Check sheet for the modelled part. Datum: model origin and axes. Units: mm. A direction names the side the tool comes from. Give positions to 0.01 mm unless a question says otherwise; leave off trailing zeros. Loops run counter-clockwise (first coordinate to the right, second up) from the corner with the lowest first, then second, coordinate; pieces in that order, holes last. Notation, with made-up numbers: (32, 24) -> (89, 24) arc R20 cw to (89, 51) -> close; hole circle Ø6 at (84, 15). An arc over 180 degrees is marked (long way). Write each question's results on one line, items separated by ' | '. Start each with the question number.
1. Mould release check, pull along X, two halves, no side actions. Record for faces 1 (the face through (-5, 3.25, 0)), 2 (the face through (-10.4, 3.6, 0)), 3 (the face through (-1.5, 0.07, -5.63)): +X half, -X half, draft (parallel to the pull), parting line (faces both ways), or undercut.
2. Cross-section at A-A on y = -2.25. Record the boundary of the cut face in (x, z), and give its area (3 significant figures).
3. Cross-section at C-C on x = -8.25. Record the boundary of the cut face in (y, z), and give its area (3 significant figures).
4. Gauge pin test, flat ends, axial feed: pin 1 Ø0.8 at (y, z) = (3.5, -2) entering from +X; pin 2 Ø0.8 at (x, z) = (1, -6) entering from +Y. Record the tip position at first contact, or that the pin passes through.
5. Cross-section at D-D on z = 3.5. Record the boundary of the cut face in (x, y).
6. Material ranges on L1, parallel to Z at x = -4.25, y = 1.75; L2, parallel to X at y = 0, z = 5.7; L3, parallel to Y at x = -6.5, z = -0.5, recorded low to high. Write a range as from..to.
7. Tool access check on faces 4 (the face through (-3, -1, -5.25)), 5 (the face through (0.1, 3.6, -0.1)), 6 (the face through (-3, 0, 6)). Record the directions out of +Z, -Z, +X, -X, +Y, -Y that give a thin tool (end or side, any length) a straight path to the whole face; none if there is none.
8. Cross-section at B-B on y = 0. Record the boundary of the cut face in (x, z).
from build123d import *

# Parameters (mm, degrees)
SKETCH1_R               = 1.5
BOSS_EXTRUDE1_DEPTH     = 6
FILLET1_R               = 1
CUT_EXTRUDE2_DEPTH      = 13.655433616
CUT_EXTRUDE2_DEPTH_BACK = 13.655433616
CUT_EXTRUDE3_DEPTH      = 16.748015748
CUT_EXTRUDE3_DEPTH_BACK = 3.5


with BuildPart() as part:
    # Sketch1 → Boss-Extrude1 (new, symmetric)
    with BuildSketch(Plane.XY):
        Polygon((-10.4, -3), (-0.7, -3), (-0.55, -4), (3.6, -3.7), (3.6, 4), (-10.4, 4), align=None)
        Circle(SKETCH1_R, mode=Mode.SUBTRACT)
    extrude(amount=BOSS_EXTRUDE1_DEPTH, both=True)

    # Fillet1
    fillet1_edges = [part.edges().sort_by_distance(p)[0] for p in [
        (-3.4, 4, -6),
        (-3.4, 4, 6),
    ]]
    fillet(fillet1_edges, radius=FILLET1_R)

    # Sketch2 → Cut-Extrude2 (cut, two sides: drawn at the far end of the back side and taken through both)
    with BuildSketch(Plane(origin=(0, 0, 0), x_dir=(0, 0, -1), z_dir=(1, 0, 0)).offset(-CUT_EXTRUDE2_DEPTH_BACK)):
        with BuildLine():
            Line((-5.25, 3), (-5.25, -4))
            Line((-5.25, -4), (5.25, -4))
            Line((5.25, -4), (5.25, 3))
            ThreePointArc((5.25, 3), (5.176776695, 3.176776695), (5, 3.25))
            Line((5, 3.25), (-5, 3.25))
            ThreePointArc((-5, 3.25), (-5.176776695, 3.176776695), (-5.25, 3))
        make_face()
    extrude(amount=CUT_EXTRUDE2_DEPTH + CUT_EXTRUDE2_DEPTH_BACK, mode=Mode.SUBTRACT)

    # Sketch3 → Cut-Extrude3 (cut, two sides: drawn at the far end of the back side and taken through both)
    with BuildSketch(Plane(origin=(3.6, 0, 0), x_dir=(0, 0, -1), z_dir=(1, 0, 0)).offset(-CUT_EXTRUDE3_DEPTH_BACK)):
        with BuildLine():
            Line((-5, 4), (5, 4))
            ThreePointArc((5, 4), (5.707106781, 3.707106781), (6, 3))
            Line((6, 3), (-6, 3))
            ThreePointArc((-6, 3), (-5.707106781, 3.707106781), (-5, 4))
        make_face()
    extrude(amount=CUT_EXTRUDE3_DEPTH + CUT_EXTRUDE3_DEPTH_BACK, mode=Mode.SUBTRACT)


solid = part.part
Geometry says:
1) face 1: draft | face 2: -X half | face 3: undercut
2) outline: (-10.4, -6) -> (3.6, -6) -> (3.6, -5.25) -> (-10.4, -5.25) -> close; (-10.4, 5.25) -> (3.6, 5.25) -> (3.6, 6) -> (-10.4, 6) -> close | area: 21.0 mm^2
3) outline: (-3, -6) -> (3, -6) arc R1 ccw to (4, -5) -> (4, 5) arc R1 ccw to (3, 6) -> (-3, 6) -> (-3, 5.25) -> (3, 5.25) arc R0.25 cw to (3.25, 5) -> (3.25, -5) arc R0.25 cw to (3, -5.25) -> (-3, -5.25) -> close | area: 18.0 mm^2
4) pin 1: x = 0.1 | pin 2: y = 3
5) outline: (-10.4, 3.25) -> (0.1, 3.25) -> (0.1, 4) -> (-10.4, 4) -> close
6) L1: -6..-5.25, 5.25..6 | L2: -10.4..-1.5, 1.5..3.6 | L3: 3.25..4
7) face 4: +X, -X, -Y | face 5: +Z, -Z, +X, +Y | face 6: +Z, +X, -X, +Y, -Y
8) outline: (-10.4, -6) -> (-1.5, -6) -> (-1.5, -5.25) -> (-10.4, -5.25) -> close; (-10.4, 5.25) -> (-1.5, 5.25) -> (-1.5, 6) -> (-10.4, 6) -> close; (1.5, -6) -> (3.6, -6) -> (3.6, -5.25) -> (1.5, -5.25) -> close; (1.5, 5.25) -> (3.6, 5.25) -> (3.6, 6) -> (1.5, 6) -> close
